CAD build for the part. Positions are in the model's coordinates, mm. A direction names the side the tool comes from. Round coordinates to 2 decimals unless told otherwise and drop trailing zeros. Order: outer loops, then holes, each group sorted by start corner. A loop starts at its lowest first (then second) coordinate and runs counter-clockwise, first axis right, second up.
```python
from build123d import *

# Parameters (mm, degrees)
SKETCH1_W           = 50
SKETCH1_H           = 31.1
BOSS_EXTRUDE1_DEPTH = 1
SKETCH2_W           = 50
SKETCH2_H           = 31.1
SKETCH2_W_2         = 48.1
SKETCH2_H_2         = 29.2
BOSS_EXTRUDE2_DEPTH = 1
SKETCH3_W           = 3
SKETCH3_H           = 3
BOSS_EXTRUDE3_DEPTH = 3.7
SKETCH4_R           = 1.55
CUT_EXTRUDE1_DEPTH  = 1
SKETCH5_W           = 21.35
SKETCH5_H           = 3
SKETCH5_W_2         = 1
SKETCH5_H_2         = 1.4
CUT_EXTRUDE2_DEPTH  = 1
SKETCH6_W           = 1.6
SKETCH6_H           = 2
SKETCH6_W_2         = 1
SKETCH6_H_2         = 1.4
BOSS_EXTRUDE4_DEPTH = 3.3
FILLET1_R           = 2
FILLET2_R           = 1
FILLET3_R           = 1
FILLET4_R           = 1
FILLET5_R           = 0.5
FILLET6_R           = 0.5


with BuildPart() as part:
    # Sketch1 → Boss-Extrude1 (new body)
    with BuildSketch(Plane.XY):
        Rectangle(SKETCH1_W, SKETCH1_H)
    extrude(amount=BOSS_EXTRUDE1_DEPTH)

    # Sketch2 → Boss-Extrude2 (add)
    with BuildSketch(Plane.XY.offset(1)):
        Rectangle(SKETCH2_W, SKETCH2_H)
        Rectangle(SKETCH2_W_2, SKETCH2_H_2, mode=Mode.SUBTRACT)
    extrude(amount=BOSS_EXTRUDE2_DEPTH)

    # Sketch3 → Boss-Extrude3 (add)
    with BuildSketch(Plane.XY.offset(1)):
        with Locations((18.55, 12.05)):
            Rectangle(SKETCH3_W, SKETCH3_H)
        with Locations((-18.55, 12.05)):
            Rectangle(SKETCH3_W, SKETCH3_H)
        with Locations((18.55, -12.05)):
            Rectangle(SKETCH3_W, SKETCH3_H)
        with Locations((-18.55, -12.05)):
            Rectangle(SKETCH3_W, SKETCH3_H)
    extrude(amount=BOSS_EXTRUDE3_DEPTH)

    # Sketch4 → Cut-Extrude1 (cut)
    with BuildSketch(Plane.XY.offset(1)):
        with Locations((-22.03, 11.55)):
            Circle(SKETCH4_R)
        with Locations(Location((22.03, 11.55, 0), (0, 0, 180))):
            Circle(SKETCH4_R)
        with Locations(Location((-22.03, -11.55, 0), (0, 0, 180))):
            Circle(SKETCH4_R)
        with Locations((22.03, -11.55)):
            Circle(SKETCH4_R)
    extrude(amount=-CUT_EXTRUDE1_DEPTH, mode=Mode.SUBTRACT)

    # Sketch5 → Cut-Extrude2 (cut)
    with BuildSketch(Plane.XY.offset(1)):
        with Locations((-6.375, 11.35)):
            Rectangle(SKETCH5_W, SKETCH5_H)
        with Locations((-6.375, -11.35)):
            Rectangle(SKETCH5_W, SKETCH5_H)
        with Locations((-8, -4.5)):
            Rectangle(SKETCH5_W_2, SKETCH5_H_2)
    extrude(amount=-CUT_EXTRUDE2_DEPTH, mode=Mode.SUBTRACT)

    # Sketch6 → Boss-Extrude4 (add)
    with BuildSketch(Plane.XY.offset(1)):
        with Locations((-8, -4.5)):
            Rectangle(SKETCH6_W, SKETCH6_H)
        with Locations((-8, -4.5)):
            Rectangle(SKETCH6_W_2, SKETCH6_H_2, mode=Mode.SUBTRACT)
    extrude(amount=BOSS_EXTRUDE4_DEPTH)

    # Fillet1
    fillet1_edges = [part.edges().sort_by_distance(p)[0] for p in [
        (24.05, 14.6, 1.5),
        (-24.05, 14.6, 1.5),
        (-24.05, -14.6, 1.5),
        (24.05, -14.6, 1.5),
        (25, -15.55, 1),
        (-25, -15.55, 1),
        (-25, 15.55, 1),
        (25, 15.55, 1),
    ]]
    fillet(fillet1_edges, radius=FILLET1_R)

    # Fillet2
    fillet2_edges = [part.edges().sort_by_distance(p)[0] for p in [
        (-20.05, -13.55, 2.85),
        (-17.05, -13.55, 2.85),
        (-17.05, -10.55, 2.85),
        (-20.05, -10.55, 2.85),
        (20.05, 13.55, 2.85),
        (17.05, 13.55, 2.85),
        (17.05, 10.55, 2.85),
        (20.05, 10.55, 2.85),
        (-20.05, 10.55, 2.85),
        (-17.05, 10.55, 2.85),
        (-17.05, 13.55, 2.85),
        (20.05, -13.55, 2.85),
        (20.05, -10.55, 2.85),
        (17.05, -10.55, 2.85),
        (17.05, -13.55, 2.85),
        (-20.05, 13.55, 2.85),
    ]]
    fillet(fillet2_edges, radius=FILLET2_R)

    # Fillet3
    fillet3_edges = [part.edges().sort_by_distance(p)[0] for p in [
        (25, 0, 0),
        (0, -15.55, 0),
        (-25, 0, 0),
        (0, 15.55, 0),
        (-24.414213562, 14.964213562, 0),
        (24.414213562, 14.964213562, 0),
        (-24.414213562, -14.964213562, 0),
        (24.414213562, -14.964213562, 0),
    ]]
    fillet(fillet3_edges, radius=FILLET3_R)

    # Fillet4
    # the kernel refuses this fillet: 1 mm, written as the material it adds along each edge
    with BuildSketch(Plane(origin=(4.3, -9.85, 1), x_dir=(-1, 0, 0), z_dir=(0, 0, -1)), Plane(origin=(-17.05, -9.85, 1), x_dir=(0, -1, 0), z_dir=(0, 0, -1)), Plane(origin=(4.3, 12.85, 1), x_dir=(-1, 0, 0), z_dir=(0, 0, -1)), Plane(origin=(4.3, 9.85, 1), x_dir=(0, 1, 0), z_dir=(0, 0, -1))) as fillet4_piece_1:
        with BuildLine():
            CenterArc((FILLET4_R, -FILLET4_R), FILLET4_R, 90, 90)
            Line((0, -FILLET4_R), (0, 0))
            Line((0, 0), (FILLET4_R, 0))
        make_face()
    extrude(amount=1)
    with BuildSketch(Plane(origin=(4.3, -12.85, 1), x_dir=(-1, 0, 0), z_dir=(0, 0, -1)), Plane(origin=(-17.05, 9.85, 1), x_dir=(0, 1, 0), z_dir=(0, 0, -1))) as fillet4_piece_2:
        with BuildLine():
            CenterArc((FILLET4_R, FILLET4_R), FILLET4_R, 180, 90)
            Line((0, FILLET4_R), (0, 0))
            Line((0, 0), (FILLET4_R, 0))
        make_face()
    extrude(amount=1)
    with BuildSketch(Plane(origin=(-17.096060799, -12.85, 0), x_dir=(0.04601201496386327, 0.9989408863786512, 0), z_dir=(0, 0, 1))) as fillet4_piece_3:
        with BuildLine():
            CenterArc((1.047072251, -0.998940886), FILLET4_R, 92.637225371, 90)
            Line((0.048131365, -1.044952901), (-0.051762724, -1.049554103))
            Line((-0.051762724, -1.049554103), (-0.099894089, -0.004601201))
            Line((-0.099894089, -0.004601201), (0.02557896, 0.096673248))
            ThreePointArc((0.02557896, 0.096673248), (0.297200415, 0.067685678), (0.996459035, 0.099894089))
            Line((0.996459035, 0.099894089), (1.001060237, 0))
        make_face()
    extrude(amount=1)
    with BuildSketch(Plane(origin=(-17.096060799, 12.85, 0), x_dir=(1, 0, 0), z_dir=(0, 0, 1))) as fillet4_piece_4:
        with BuildLine():
            CenterArc((1.046060799, -1), FILLET4_R, 90, 90)
            Line((0.046060799, -1), (-0.053939201, -1))
            ThreePointArc((-0.053939201, -1), (-0.053939201, -0.3), (-0.09539392, -0.03))
            Line((-0.09539392, -0.03), (0, 0.1))
            Line((0, 0.1), (1.046060799, 0.1))
            Line((1.046060799, 0.1), (1.046060799, 0))
        make_face()
    extrude(amount=1)

    # Fillet5
    fillet5_edges = [part.edges().sort_by_distance(p)[0] for p in [
        (-7.2, -4.5, 1),
        (-8, -3.5, 1),
        (-8.8, -4.5, 1),
        (-8, -5.5, 1),
    ]]
    fillet(fillet5_edges, radius=FILLET5_R)

    # Fillet6
    fillet6_edges = [part.edges().sort_by_distance(p)[0] for p in [
        (-8, -5.2, 0),
        (-7.5, -4.5, 0),
        (-8, -3.8, 0),
        (-8.5, -4.5, 0),
    ]]
    fillet(fillet6_edges, radius=FILLET6_R)


solid = part.part
```
1. Mould opens along Y. For faces 1 (the face through (-25, -0.2, 1.5)), 2 (the face through (-17.335, 10.851, 2.876)) say: released by +Y, released by -Y, zero draft, split by the parting line, or undercut.
2. Drill centre lines: line 1 (Y direction, x = -0.5, z = 0.95); line 2 (X direction, y = 5.5, z = 1.8); line 3 (Y direction, x = 13, z = 1.15). Where is each one in solid material? Low to high.
3. Cut at A-A, the plane z = 3.35. Give the number of separate pieces and of enclosed holes in the cut face, and give its area (3 significant figures).
4. Tool access for faces 3 (the face through (-16.765, -12.549, 0.493)), 4 (the face through (-0.3, 14.6, 1.5)), 5 (the face through (19, 12, 4.7)): list every direction of +Z, -Z, +X, -X, +Y, -Y with a clear straight run to the whole face (end or side of a thin tool).
5. Pin check, flat tips, straight feed: P1, Ø1.5, axis at x = -12.5, y = -9, coming from the +Z side; P2, Ø1.1, axis at x = -18.5, z = 3.5, coming from the -Y side; P3, Ø0.8, axis at x = -8, z = 3.5, coming from the +Y side. Stop position of each tip, or through.
6. Cut at B-B, the plane y = -0.5. Write the cut outline in (x, z), and give its area (3 significant figures).
Outcome:
1. face 1: zero draft
1. face 2: undercut
2. line 1: y = -15.55 to -12.85, -9.85 to 9.85, 12.85 to 15.55
2. line 2: x = -25 to -24.05, 24.05 to 25
2. line 3: y = -15.55 to -14.6, 14.6 to 15.55
3. separate pieces: 5
3. enclosed holes: 1
3. area: 34.4 mm2
4. face 3: +Z, -Z
4. face 4: +Z
4. face 5: +Z, +X, -X, +Y, -Y
5. P1: stops at z = 1
5. P2: stops at y = -13.55
5. P3: stops at y = -3.5
6. outline: (-25, 1) arc R1 ccw to (-24, 0) - (24, 0) arc R1 ccw to (25, 1) - (25, 2) - (24.05, 2) - (24.05, 1) - (-24.05, 1) - (-24.05, 2) - (-25, 2) - close
6. area: 51.5 mm2
